```python
from build123d import *

# Parameters (mm, degrees)
SKETCH_1_R               = 42.5
EXTRUDE_1_DEPTH          = 40
SKETCH_2_R               = 27.5
SKETCH_2_R_2             = 8
CUT_EXTRUDE_1_DEPTH      = 35
SKETCH_3_R               = 4
CUT_EXTRUDE_2_DEPTH      = 35
PATTERN_CIRCULAR_1_COUNT = 8
CUT_EXTRUDE_START        = -2
SKETCH_4_R               = 27.5
CUT_EXTRUDE_3_DEPTH      = 2
EXTRUDE_START            = 4
SKETCH_5_R               = 8
EXTRUDE_2_DEPTH          = 4
FILLET_1_R               = 3


with BuildPart() as part:
    # Эскиз1 → Бобышка-Вытянуть1 (new body)
    with BuildSketch(Plane(origin=(0, 0, 0), x_dir=(1, 0, 0), z_dir=(0, 1, 0))):
        with Locations(Location((0, 0, 0), (0, 0, 270))):
            Circle(SKETCH_1_R)
    extrude(amount=EXTRUDE_1_DEPTH)

    # Эскиз2 → Вырез-Вытянуть1 (cut)
    with BuildSketch(Plane(origin=(0, 40, 0), x_dir=(1, 0, 0), z_dir=(0, 1, 0))):
        with Locations(Location((0, 0, 0), (0, 0, 270))):
            Circle(SKETCH_2_R)
        with Locations(Location((0, 0, 0), (0, 0, 270))):
            Circle(SKETCH_2_R_2, mode=Mode.SUBTRACT)
    extrude(amount=-CUT_EXTRUDE_1_DEPTH, mode=Mode.SUBTRACT)

    # Эскиз3 → Вырез-Вытянуть2 (cut)
    with BuildSketch(Plane(origin=(0, 5, 0), x_dir=(1, 0, 0), z_dir=(0, 1, 0))):
        with Locations(Location((0, 17.75, 0), (0, 0, 270))):
            Circle(SKETCH_3_R)
    cut_extrude_2 = extrude(amount=-CUT_EXTRUDE_2_DEPTH, mode=Mode.SUBTRACT)

    # Круговой массив1: Вырез-Вытянуть2 ×8 about axis
    pattern_circular_1_axis = Axis((0, 0, 0), (0, 1, 0))
    for i in range(1, PATTERN_CIRCULAR_1_COUNT):
        add(cut_extrude_2.rotate(pattern_circular_1_axis, i * 360 / PATTERN_CIRCULAR_1_COUNT), mode=Mode.SUBTRACT)

    # Эскиз4 → Вырез-Вытянуть3 (cut)
    with BuildSketch(Plane.XZ.offset(CUT_EXTRUDE_START)):
        with Locations(Location((0, 0, 0), (0, 0, 90))):
            Circle(SKETCH_4_R)
    extrude(amount=CUT_EXTRUDE_3_DEPTH, mode=Mode.SUBTRACT)

    # Эскиз5 → Бобышка-Вытянуть2 (add)
    with BuildSketch(Plane(origin=(0, 40, 0), x_dir=(1, 0, 0), z_dir=(0, 1, 0)).offset(EXTRUDE_START)):
        with Locations(Location((0, 0, 0), (0, 0, 270))):
            Circle(SKETCH_5_R)
    extrude(amount=-EXTRUDE_2_DEPTH)

    # Скругление1
    fillet_1_edges = [part.edges().sort_by_distance(p)[0] for p in [
        (0, 0, -42.5),
        (0, 40, -42.5),
    ]]
    fillet(fillet_1_edges, radius=FILLET_1_R)


solid = part.part
```
Could you check a few things on this model? Use its own coordinates, in mm. A direction names the side the tool comes from. Round coordinates to 2 decimals unless told otherwise and drop trailing zeros. Loops run counter-clockwise (first coordinate to the right, second up) from the corner with the lowest first, then second, coordinate; pieces in that order, holes last. Notation, with made-up numbers: M 45,33 L 49,33 A29 cw 49,68 Z; hole C 73,37 d5. An arc over 180 degrees is marked long. Answer as CSV lines item,"result".
1) Which directions (+Z, -Z, +X, -X, +Y, -Y) give clear straight access to the entire face, cutting with the end or side of a thin tool? Please do faces 1 (the cylindrical face through (10.403, 3.521, -15.925)), 2 (the cylindrical face through (-7.81, 24.77, -1.73)), 3 (the cylindrical face through (24.397, 1.014, 12.69)).
From the geometry:
face 1,"+Y, -Y"
face 2,"+Y"
face 3,"-Y"
2) Imagine slicing it at A-A on x = 0. List the corners of the cut face in (y, z) for me.
From the geometry:
outline,"M 0,-39.5 A3 ccw 3,-42.5 L 37,-42.5 A3 ccw 40,-39.5 L 40,-27.5 L 5,-27.5 L 5,-21.75 L 2,-21.75 L 2,-27.5 L 0,-27.5 Z; M 0,27.5 L 2,27.5 L 2,21.75 L 5,21.75 L 5,27.5 L 40,27.5 L 40,39.5 A3 ccw 37,42.5 L 3,42.5 A3 ccw 0,39.5 Z; M 2,-13.75 L 5,-13.75 L 5,-8 L 44,-8 L 44,8 L 5,8 L 5,13.75 L 2,13.75 Z"
3) Imagine slicing it at D-D on x = 15. Count the separate pieces of the cut face and the enclosed holes in it, and give its area (3 significant figures).
From the geometry:
separate pieces,"4"
enclosed holes,"0"
area,"1,410 mm^2"
4) We'd pull the mould along Z, two halves only. Please class faces 4 (the flat face through (0, 2, 0)), 5 (the flat face through (27, 40, 8)), 6 (the cylindrical face through (-25.861, 19.762, -33.727)): released by +Z, released by -Z, zero draft, split by the parting line, or undercut.
From the geometry:
face 4,"undercut"
face 5,"zero draft"
face 6,"split by the parting line"
5) Imagine slicing it at B-B on z = 0. List the corners of the cut face in (x, y) for me.
From the geometry:
outline,"M -42.5,3 A3 ccw -39.5,0 L -27.5,0 L -27.5,2 L -21.75,2 L -21.75,5 L -27.5,5 L -27.5,40 L -39.5,40 A3 ccw -42.5,37 Z; M -13.75,2 L 13.75,2 L 13.75,5 L 8,5 L 8,44 L -8,44 L -8,5 L -13.75,5 Z; M 21.75,2 L 27.5,2 L 27.5,0 L 39.5,0 A3 ccw 42.5,3 L 42.5,37 A3 ccw 39.5,40 L 27.5,40 L 27.5,5 L 21.75,5 Z"
6) Imagine slicing it at C-C on y = 16.5. List the corners of the cut face in (x, z) for me.
From the geometry:
outline,"C 0,0 d85; C 0,0 d16; hole C 0,0 d55"
7) For pin 1 Ø1 at (x, y) = (6.5, 14.5) entering from -Z; pin 2 Ø6.5 at (x, z) = (-12.55, 12.55) entering from +Y; pin 3 Ø16.5 at (x, z) = (-2, 10.5) entering from -Y; pin 4 Ø4 at (y, z) = (5.5, -13) entering from -X, each with a flat end and sliding along its axis, tell me the tip position at first contact or that it passes through.
From the geometry:
pin 1,"z = -42.07"
pin 2,"through"
pin 3,"y = 2"
pin 4,"x = -41.05"
8) If I drill on probe 1 along X at (y, z) = (10.5, -2.5); probe 2 along Z at (x, y) = (-6.5, 20); probe 3 along Y at (x, z) = (-8, 15), over which ranges is the centre line in solid material (lowest first)?
From the geometry:
probe 1,"-42.43 to -27.39, -7.6 to 7.6, 27.39 to 42.43"
probe 2,"-42 to -26.72, -4.66 to 4.66, 26.72 to 42"
probe 3,"2 to 5"
